Could you check a few things on this model? Use its own coordinates, in mm. A direction names the side the tool comes from. Round coordinates to 2 decimals unless told otherwise and drop trailing zeros. Loops run counter-clockwise (first coordinate to the right, second up) from the corner with the lowest first, then second, coordinate; pieces in that order, holes last. Notation, with made-up numbers: (-11, 65.25) - (2, 65.25) arc R4 cw to (2, 70.25) - close; hole circle Ø8 at (29, 21). An arc over 180 degrees is marked (long way). Answer as CSV lines item,"result". Start each with the question number.
1) Please list where these lines run through material, in increasing order: line 1 along Z through (x, y) = (11, 3.25); line 2 along X through (y, z) = (3, -0.25) (3 decimals); line 3 along X through (y, z) = (5, 0) (3 decimals).
2) I'm going to push flat-ended pins straight in: pin 1 Ø1.9 at (y, z) = (6.5, -1.5) entering from +X; pin 2 Ø8 at (x, z) = (0, 8.5) entering from +Y. Where does each tip first touch, or does it pass through?
3) Suppose I cut it at C-C, the plane y = 1.5. Write out the boundary of the cut face in (x, z) (3 decimals).
4) We'd pull the mould along X, two halves only. Please class faces 4 (the face through (-5, 3, 12.7)), 5 (the face through (-3.41, 1.93, 6.39)), 6 (the face through (18.904, 1.932, 6.314)), 7 (the face through (22.225, 2, 0)): pulls with the +X half, pulls with the -X half, needs draft (parallel to the pull), parting line crosses it, or undercut.
5) Suppose I cut it at D-D, the plane x = 18. Write out the boundary of the cut face in (y, z).
6) Which directions (+Z, -Z, +X, -X, +Y, -Y) give clear straight access to the entire face, cutting with the end or side of a thin tool? Please do faces 1 (the face through (-16, 7.62, 0)), 2 (the face through (8, 2, 7.982)), 3 (the face through (8, 3.81, 0)).
7) Suppose I cut it at A-A, the plane z = -6.35. Write out the boundary of the cut face in (x, y) (3 decimals).
8) Suppose I cut it at B-B, the plane x = -10. Write out the boundary of the cut face in (y, z), then the cut area to 3 significant figures.
```python
from build123d import *

# Parameters (mm, degrees)
BOSS_EXTRUDE1_DEPTH = 12.7
SKETCH2_R           = 3.81
CUT_EXTRUDE1_DEPTH  = 8.62


with BuildPart() as part:
    # Sketch1 → Boss-Extrude1 (new body, symmetric)
    with BuildSketch(Plane.XY):
        Polygon((-22.225, 7.62), (-6.731, 7.62), (-6.731, 3.81), (22.225, 3.81), (22.225, 0), (-22.225, 0), align=None)
    extrude(amount=BOSS_EXTRUDE1_DEPTH, both=True)

    # Sketch2 → Cut-Extrude1 (cut, through all)
    with BuildSketch(Plane(origin=(0, 7.62, 0), x_dir=(1, 0, 0), z_dir=(0, 1, 0))):
        with Locations((-11.811, 0)):
            Circle(SKETCH2_R)
        with BuildLine():
            Line((-1.778, 7.98195), (17.272, 7.98195))
            ThreePointArc((17.272, 7.98195), (18.90395, 6.35), (17.272, 4.71805))
            Line((17.272, 4.71805), (-1.778, 4.71805))
            ThreePointArc((-1.778, 4.71805), (-3.40995, 6.35), (-1.778, 7.98195))
        make_face()
        with BuildLine():
            Line((-1.778, -4.71805), (17.272, -4.71805))
            ThreePointArc((17.272, -4.71805), (18.90395, -6.35), (17.272, -7.98195))
            Line((17.272, -7.98195), (-1.778, -7.98195))
            ThreePointArc((-1.778, -7.98195), (-3.40995, -6.35), (-1.778, -4.71805))
        make_face()
    extrude(amount=-CUT_EXTRUDE1_DEPTH, mode=Mode.SUBTRACT)


solid = part.part
```
Filled sheet:
1,line 1,"-12.7 to -7.98, -4.72 to 4.72, 7.98 to 12.7"
1,line 2,"-22.225 to -15.613, -8.009 to 22.225"
1,line 3,"-22.225 to -15.621, -8.001 to -6.731"
2,pin 1,"x = -6.73"
2,pin 2,"y = 3.81"
3,outline,"(-22.225, -12.7) - (22.225, -12.7) - (22.225, 12.7) - (-22.225, 12.7) - close; hole circle Ø7.62 at (-11.811, 0); hole (-1.778, -7.982) - (17.272, -7.982) arc R1.632 ccw to (17.272, -4.718) - (-1.778, -4.718) arc R1.632 ccw to start; hole (-1.778, 4.718) - (17.272, 4.718) arc R1.632 ccw to (17.272, 7.982) - (-1.778, 7.982) arc R1.632 ccw to start"
4,face 4,"needs draft"
4,face 5,"undercut"
4,face 6,"undercut"
4,face 7,"pulls with the +X half"
5,outline,"(0, -12.7) - (3.81, -12.7) - (3.81, -7.81) - (0, -7.81) - close; (0, -4.89) - (3.81, -4.89) - (3.81, 4.89) - (0, 4.89) - close; (0, 7.81) - (3.81, 7.81) - (3.81, 12.7) - (0, 12.7) - close"
6,face 1,"+Z, -Z, +X, -X, +Y"
6,face 2,"+Y, -Y"
6,face 3,"+Z, -Z, +X, +Y"
7,outline,"(-22.225, 0) - (-3.41, 0) - (-3.41, 3.81) - (-6.731, 3.81) - (-6.731, 7.62) - (-22.225, 7.62) - close; (18.904, 0) - (22.225, 0) - (22.225, 3.81) - (18.904, 3.81) - close"
8,outline,"(0, -12.7) - (7.62, -12.7) - (7.62, -3.35) - (0, -3.35) - close; (0, 3.35) - (7.62, 3.35) - (7.62, 12.7) - (0, 12.7) - close"
8,area,"142 mm²"
